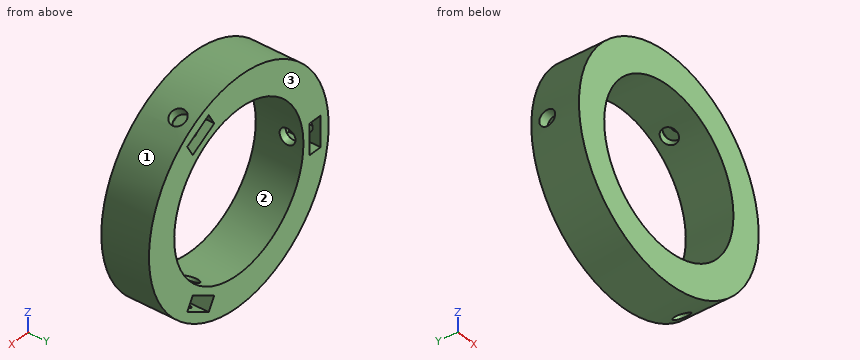
from build123d import *

# Parameters (mm, degrees)
SKETCH1_R           = 21
SKETCH1_R_2         = 15.1
BOSS_EXTRUDE1_DEPTH = 9
SKETCH2_W           = 2.6
SKETCH2_H           = 5.8
CUT_EXTRUDE1_DEPTH  = 6
SKETCH3_R           = 1.5
CUT_EXTRUDE2_DEPTH  = 6
CIRPATTERN1_COUNT   = 3


with BuildPart() as part:
    # Sketch1 → Boss-Extrude1 (new body)
    with BuildSketch(Plane(origin=(0, 0, 0), x_dir=(1, 0, 0), z_dir=(0, 1, 0))):
        with Locations(Location((0, 0, 0), (0, 0, 270))):
            Circle(SKETCH1_R)
        with Locations(Location((0, 0, 0), (0, 0, 270))):
            Circle(SKETCH1_R_2, mode=Mode.SUBTRACT)
    extrude(amount=BOSS_EXTRUDE1_DEPTH)

    # Sketch2 → Cut-Extrude1 (cut)
    with BuildSketch(Plane(origin=(0, 9, 0), x_dir=(1, 0, 0), z_dir=(0, 1, 0))):
        with Locations((-17.8, 0)):
            Rectangle(SKETCH2_W, SKETCH2_H)
    cut_extrude1 = extrude(amount=-CUT_EXTRUDE1_DEPTH, mode=Mode.SUBTRACT)

    # Sketch3 → Cut-Extrude2 (cut, symmetric)
    with BuildSketch(Plane.ZY.offset(16.5)):
        with Locations(Location((0, 6, 0), (0, 0, 180))):
            Circle(SKETCH3_R)
    cut_extrude2 = extrude(amount=CUT_EXTRUDE2_DEPTH, both=True, mode=Mode.SUBTRACT)

    # CirPattern1: Cut-Extrude1, Cut-Extrude2 ×3 about axis
    cirpattern1_axis = Axis((0, 0, 0), (0, 1, 0))
    add([cut_extrude1.rotate(cirpattern1_axis, i * 360 / CIRPATTERN1_COUNT) for i in range(1, CIRPATTERN1_COUNT)], mode=Mode.SUBTRACT)
    add([cut_extrude2.rotate(cirpattern1_axis, i * 360 / CIRPATTERN1_COUNT) for i in range(1, CIRPATTERN1_COUNT)], mode=Mode.SUBTRACT)


solid = part.part
Input: part model. Units: mm. Frame: model coordinates. Face numbers are marked on the shaded views. Give positions to 0.01 mm unless a question says otherwise; leave off trailing zeros. Write each loop counter-clockwise with the first axis right and the second up, starting at its lowest first coordinate (ties: lowest second). Pieces come first, ordered by that corner, then holes. Notation, with made-up numbers: M 60.5,7.25 L 96.5,7.25 A27 cw 96.5,42.25 Z; hole C 2.5,12 d6. An arc over 180 degrees is marked long. Write item = value, one per line. Start each with the question number.
1) Draft query along Z for the marked faces 1, 2 and 3. Return one class per face: +Z half, -Z half, draft (parallel to the pull), parting line (faces both ways), or undercut.
2) Cut plane A-A on z = 0. Return the cut outline in (x, y), then the cut area to 3 significant figures.
3) Material intervals for line 1 along X through (y, z) = (7, -1.5); line 2 along Y through (x, z) = (-19.6, 0); line 3 along X through (y, z) = (8.25, 2.5), sorted ascending. Write a range as [from, to].
4) Cut plane C-C on y = 3.5. Return the cut outline in (x, z).
5) Cut plane D-D on z = 11.5. Return the cut outline in (x, y).
6) Cut plane B-B on x = 0. Return the cut outline in (y, z).
7) First-contact query: pin 1 Ø1.8 at (y, z) = (6, 0) entering from -X; pin 2 Ø1 at (y, z) = (2, -5) entering from -X; pin 3 Ø1.3 at (x, y) = (-18, 5) entering from +Z. Flat tips, straight axial feed; report the tip coordinate or a pass-through.
Solved:
q1.face_1 = parting line
q1.face_2 = undercut
q1.face_3 = draft
q2.outline = M -21,0 L -15.1,0 L -15.1,4.5 L -16.5,4.5 L -16.5,3 L -19.1,3 L -19.1,4.5 L -21,4.5 Z; M -21,7.5 L -19.1,7.5 L -19.1,9 L -21,9 Z; M -16.5,7.5 L -15.1,7.5 L -15.1,9 L -16.5,9 Z; M 15.1,0 L 21,0 L 21,9 L 15.1,9 Z
q2.area = 80.7 mm2
q3.line_1 = [-20.95, -19.1], [-16.5, -15.03], [15.03, 20.95]
q3.line_2 = [0, 4.5], [7.5, 9]
q3.line_3 = [-20.85, -19.1], [-16.5, -14.89], [14.89, 20.85]
q4.outline = C 0,0 d42; hole M -19.1,-2.9 L -16.5,-2.9 L -16.5,2.9 L -19.1,2.9 Z; hole C 0,0 d30.2; hole M 5.74,-15.74 L 7.04,-17.99 L 12.06,-15.09 L 10.76,-12.84 Z; hole M 5.74,15.74 L 10.76,12.84 L 12.06,15.09 L 7.04,17.99 Z
q5.outline = M -17.57,0 L -9.79,0 L -9.79,9 L -17.57,9 Z; M 9.79,0 L 17.57,0 L 17.57,9 L 9.79,9 Z
q6.outline = M 0,-21 L 9,-21 L 9,-15.1 L 0,-15.1 Z; M 0,15.1 L 9,15.1 L 9,21 L 0,21 Z
q7.pin_1 = 15.07
q7.pin_2 = -20.51
q7.pin_3 = 11.83
